CAD build for the part. Positions are in the model's coordinates, mm. A direction names the side the tool comes from. Give positions to 0.01 mm unless a question says otherwise; leave off trailing zeros. Write each loop counter-clockwise with the first axis right and the second up, starting at its lowest first coordinate (ties: lowest second). Pieces come first, ordered by that corner, then holes. Notation, with made-up numbers: (10.25, 7.25) -> (17.25, 7.25) arc R25 ccw to (17.25, 28.25) -> close; hole circle Ø9 at (55.25, 52.5). An arc over 180 degrees is marked (long way). Answer as a JSON object with one key per item and string values.
```python
from build123d import *

# Parameters (mm, degrees)
SKETCH1_R           = 30
BOSS_EXTRUDE1_DEPTH = 500
SKETCH2_R           = 25
CUT_EXTRUDE1_DEPTH  = 100
SKETCH3_W           = 100
SKETCH3_H           = 100
BOSS_EXTRUDE2_DEPTH = 15


with BuildPart() as part:
    # Sketch1 → Boss-Extrude1 (new body)
    with BuildSketch(Plane(origin=(0, 0, 0), x_dir=(1, 0, 0), z_dir=(0, 1, 0))):
        with Locations(Location((0, 0, 0), (0, 0, 270))):
            Circle(SKETCH1_R)
    extrude(amount=BOSS_EXTRUDE1_DEPTH)

    # Sketch2 → Cut-Extrude1 (cut)
    with BuildSketch(Plane(origin=(0, 0, 0), x_dir=(-1, 0, 0), z_dir=(0, -1, 0))):
        with Locations(Location((0, 0, 0), (0, 0, 90))):
            Circle(SKETCH2_R)
    extrude(amount=-CUT_EXTRUDE1_DEPTH, mode=Mode.SUBTRACT)

    # Sketch3 → Boss-Extrude2 (add)
    with BuildSketch(Plane(origin=(0, 500, 0), x_dir=(1, 0, 0), z_dir=(0, 1, 0))):
        Rectangle(SKETCH3_W, SKETCH3_H)
    extrude(amount=BOSS_EXTRUDE2_DEPTH)


solid = part.part
```
1) Slice it at B-B (y = 46.5). List the corners of the cut face in (x, z), then the cut area to 3 significant figures.
Model answer:
{"outline": "circle Ø60 at (0, 0); hole circle Ø50 at (0, 0)", "area": "864 mm2"}
2) Slice it at D-D (y = 148). List the corners of the cut face in (x, z).
Model answer:
{"outline": "circle Ø60 at (0, 0)"}
3) 3-axis set-ups, long thin cutter, end or side, ignore diameter. For faces 1 (the flat face through (-1, 515, -1)), 2 (the cylindrical face through (1.32, 246.5, -29.97)): which of +Z, -Z, +X, -X, +Y, -Y reach the whole face in a straight line?
Model answer:
{"face 1": "+Z, -Z, +X, -X, +Y", "face 2": "-Y"}
4) Wall check: probe 1 along X at (y, z) = (73, 0); probe 2 along Y at (x, z) = (37, 26); probe 3 along Y at (x, z) = (16.5, 12.5). Give the ranges that are in metal, low to high.
Model answer:
{"probe 1": "x = -30 to -25, 25 to 30", "probe 2": "y = 500 to 515", "probe 3": "y = 100 to 515"}
5) Pin check, flat tip, straight feed: pin 1 (4 mm diameter, centred on x = 13, z = -30.5, fed in from -Y). Stop position of the tip, or through.
Model answer:
{"pin 1": "stops at y = 500"}
6) Mould opens along X. For faces 3 (the flat face through (-1, 507, 50)), 4 (the flat face through (50, 507, 1)), 5 (the cylindrical face through (7.509, 49.3, -23.846)) say: released by +X, released by -X, zero draft, split by the parting line, or undercut.
Model answer:
{"face 3": "zero draft", "face 4": "released by +X", "face 5": "undercut"}
7) Slice it at C-C (z = 0). List the corners of the cut face in (x, y), then the cut area to 3 significant figures.
Model answer:
{"outline": "(-50, 500) -> (-30, 500) -> (-30, 0) -> (-25, 0) -> (-25, 100) -> (25, 100) -> (25, 0) -> (30, 0) -> (30, 500) -> (50, 500) -> (50, 515) -> (-50, 515) -> close", "area": "26,500 mm2"}
8) Slice it at A-A (x = 0). List the corners of the cut face in (y, z), then the cut area to 3 significant figures.
Model answer:
{"outline": "(0, -30) -> (500, -30) -> (500, -50) -> (515, -50) -> (515, 50) -> (500, 50) -> (500, 30) -> (0, 30) -> (0, 25) -> (100, 25) -> (100, -25) -> (0, -25) -> close", "area": "26,500 mm2"}
